Check sheet for the modelled part. Datum: model origin and axes. Units: mm. A direction names the side the tool comes from. Give positions to 0.01 mm unless a question says otherwise; leave off trailing zeros. Order: outer loops, then holes, each group sorted by start corner. A loop starts at its lowest first (then second) coordinate and runs counter-clockwise, first axis right, second up.
```python
from build123d import *

# Parameters (mm, degrees)
F0_W     = 100
F0_H     = 100
F1_DEPTH = 100
F3_R     = 15
F4_DEPTH = 30
F2_R     = 15
F5_DEPTH = 30
F6_W     = 100
F6_H     = 100
F7_DEPTH = 25.4
F9_D     = 30


with BuildPart() as f1:
    # F0 (on Front) → F1 (new body)
    with BuildSketch(Plane.XZ):
        with Locations((50, 50)):
            Rectangle(F0_W, F0_H)
    extrude(amount=F1_DEPTH)

    # F3 (on face) → F4 (join)
    with BuildSketch(Plane(origin=(0, 0, 0), x_dir=(1, 0, 0), z_dir=(0, 0, -1))):
        with Locations((50.003275, 44.529211)):
            Circle(F3_R)
    extrude(amount=F4_DEPTH)

    # F2 (on face) → F5 (join)
    with BuildSketch(Plane.XY.offset(100)):
        with Locations((49.247686, -49.222711)):
            Circle(F2_R)
    extrude(amount=F5_DEPTH)

    # F6 (on face) → F7 (join)
    with BuildSketch(Plane(origin=(0, 0, 0), x_dir=(-1, 0, 0), z_dir=(0, 1, 0))):
        with Locations((-50, 50)):
            Rectangle(F6_W, F6_H)
    extrude(amount=F7_DEPTH)

    # F9 (through all)
    with Locations(Plane(origin=(0, 25.4, 0), x_dir=(-1, 0, 0), z_dir=(0, 1, 0))):
        with Locations((-50.120577, 51.322706)):
            Hole(F9_D / 2)


solid = f1.part
```
(1) Sectioned sample at B-B (y = -36.5). Enter the section's corners in (x, z).
(2) Sectioned sample at A-A (x = 57). Enter the section's corners in (y, z).
(3) Release check for a two-part mould opening along Z. For faces 1 (the face through (62, -38, 100)), 2 (the face through (48.05, -59.4, -14.79)), 3 (the face through (39.1, -38.2, 61.5)) record: released by +Z, released by -Z, zero draft, split by the parting line, or undercut.
(4) Sectioned sample at C-C (z = 64.5). Enter the section's corners in (x, y).
(5) Tool access check on faces 4 (the face through (56.17, -62.53, 114.79)), 5 (the face through (38, -100, 40)). Record the directions out of +Z, -Z, +X, -X, +Y, -Y that give a thin tool (end or side, any length) a straight path to the whole face; none if there is none.
(6) Thickness scan on L1, parallel to Z at x = 76.5, y = -29; L2, parallel to X at y = -7, z = 48; L3, parallel to Z at x = 43, y = -56. Record the ranges inside material, lowest first.
(7) Sectioned sample at D-D (y = 1.5). Enter the section's corners in (x, z), plus the area to 3 significant figures.
(8) Go/stop test with flat-tipped pins: P1, Ø1, axis at x = 78, y = -50.5, coming from the -Z side; P2, Ø10, axis at x = 70, y = -84, coming from the +Z side; P3, Ø5, axis at y = -50.5, z = 106.5, coming from the +X side. Record where each tip stops, or that it passes through.
Values follow:
1. outline: (0, 0) - (37.33, 0) - (37.33, -30) - (62.67, -30) - (62.67, 0) - (100, 0) - (100, 100) - (57.19, 100) - (57.19, 130) - (41.3, 130) - (41.3, 100) - (0, 100) - close; hole circle Ø30 at (50.12, 51.32)
2. outline: (-100, 0) - (-57.8, 0) - (-57.8, -30) - (-31.26, -30) - (-31.26, 0) - (25.4, 0) - (25.4, 37.99) - (-100, 37.99) - close; (-100, 64.65) - (25.4, 64.65) - (25.4, 100) - (-36.38, 100) - (-36.38, 130) - (-62.06, 130) - (-62.06, 100) - (-100, 100) - close
3. face 1: released by +Z
3. face 2: zero draft
3. face 3: undercut
4. outline: (0, -100) - (42.95, -100) - (42.95, 25.4) - (0, 25.4) - close; (57.29, -100) - (100, -100) - (100, 25.4) - (57.29, 25.4) - close
5. face 4: +Z
5. face 5: +Z, -Z, +X, -X, -Y
6. L1: z = 0 to 100
6. L2: x = 0 to 35.49, 64.75 to 100
6. L3: z = -30 to 38.12, 64.52 to 130
7. outline: (0, 0) - (100, 0) - (100, 100) - (0, 100) - close; hole circle Ø30 at (50.12, 51.32)
7. area: 9,290 mm2
8. P1: stops at z = 0
8. P2: stops at z = 100
8. P3: stops at x = 64.25
